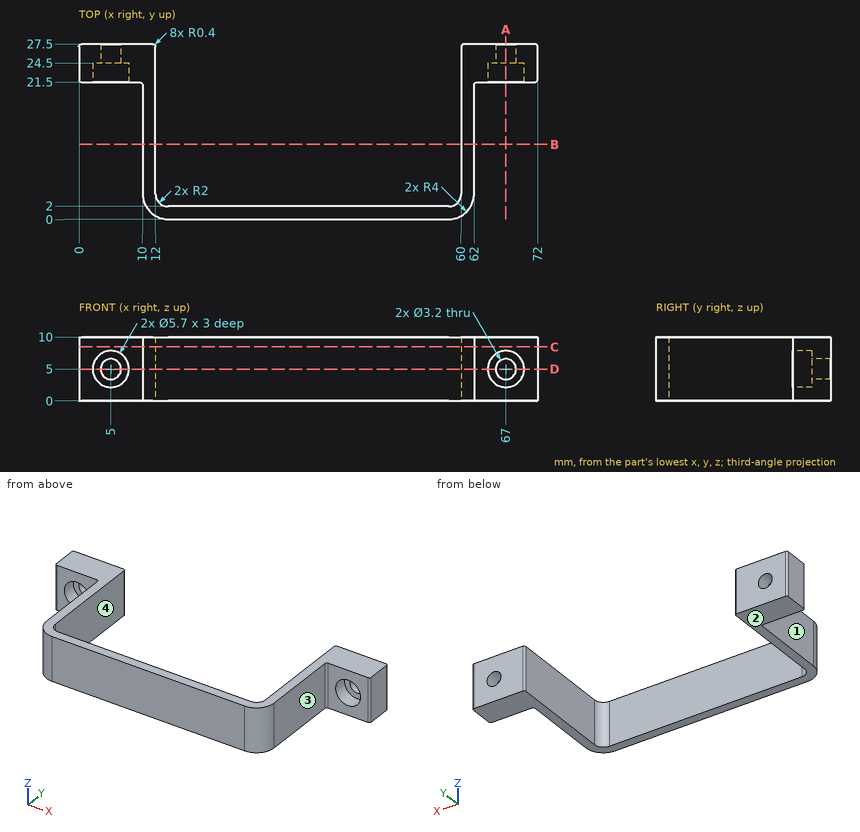
Can you work these out from the drawing? Everything is in mm from the part's minimum corner. A direction names the side the tool comes from. Give positions to 0.01 mm unless a question says otherwise; leave off trailing zeros. Order: outer loops, then holes, each group sorted by start corner. A loop starts at its lowest first (then second) coordinate and runs counter-clockwise, first axis right, second up.
1. Suppose I cut it at C-C (z = 8.5). List the corners of the cut face in (x, y) for me, plus the area to 3 significant figures.
2. Suppose I cut it at B-B (y = 11.75). List the corners of the cut face in (x, z) for me.
3. Will these pins go through, and if not, where does the flat tip stop? P1, Ø3, axis at y = 15.5, z = 5, coming from the -X side; P2, Ø5, axis at x = 67, z = 5, coming from the -Y side; P3, Ø5, axis at y = 6, z = 4.5, coming from the +X side.
4. For the marked faces 1, 2, 3 and 4, which set-ups out of +Z, -Z, +X, -X, +Y, -Y let a thin tool reach every point of the face, with its end or its side?
5. I need wall thicknesses on L1, parallel to X at y = 15.5, z = 5.75; L2, parallel to X at y = 25.75, z = 8.25; L3, parallel to Z at x = 5, y = 26.05. Which ranges of each line are inside material? Lowest first, please.
6. Suppose I cut it at A-A (x = 67). List the corners of the cut face in (y, z) for me, plus the area to 3 significant figures.
7. Suppose I cut it at D-D (z = 5). Give the number of separate pieces and of enclosed holes in the cut face, plus the area to 3 significant figures.
Solved:
1. outline: (0, 21.9) arc R0.4 ccw to (0.4, 21.5) - (9.6, 21.5) arc R0.4 cw to (10, 21.1) - (10, 4) arc R4 ccw to (14, 0) - (58, 0) arc R4 ccw to (62, 4) - (62, 21.1) arc R0.4 cw to (62.4, 21.5) - (71.6, 21.5) arc R0.4 ccw to (72, 21.9) - (72, 27.1) arc R0.4 ccw to (71.6, 27.5) - (60.4, 27.5) arc R0.4 ccw to (60, 27.1) - (60, 4) arc R2 cw to (58, 2) - (14, 2) arc R2 cw to (12, 4) - (12, 27.1) arc R0.4 ccw to (11.6, 27.5) - (0.4, 27.5) arc R0.4 ccw to (0, 27.1) - close
1. area: 321 mm2
2. outline: (10, 0) - (12, 0) - (12, 10) - (10, 10) - close; (60, 0) - (62, 0) - (62, 10) - (60, 10) - close
3. P1: stops at x = 10
3. P2: stops at y = 24.5
3. P3: stops at x = 62
4. face 1: +Z, -Z, -X, -Y
4. face 2: -Z, +X, -X, +Y, -Y
4. face 3: +Z, -Z, +X, -Y
4. face 4: +Z, -Z, +Y
5. L1: x = 10 to 12, 60 to 62
5. L2: x = 0 to 12, 60 to 72
5. L3: z = 0 to 3.4, 6.6 to 10
6. outline: (21.5, 0) - (27.5, 0) - (27.5, 3.4) - (24.5, 3.4) - (24.5, 2.15) - (21.5, 2.15) - close; (21.5, 7.85) - (24.5, 7.85) - (24.5, 6.6) - (27.5, 6.6) - (27.5, 10) - (21.5, 10) - close
6. area: 33.3 mm2
7. separate pieces: 3
7. enclosed holes: 0
7. area: 267 mm2
